Study the drawing (mm; zero at the part's minimum x, y, z) and answer. Round coordinates to 2 decimals unless told otherwise and drop trailing zeros. Order: outer loops, then holes, each group sorted by start corner. A loop starts at its lowest first (then second) coordinate and runs counter-clockwise, first axis right, second up. Notation, with made-up numbers: (-15.5, 6.5) - (14.5, 6.5) arc R23 cw to (14.5, 32.5) - close; hole circle Ø5 at (33.5, 1). An arc over 180 degrees is marked (long way). Put each result on its own line as item: value. Start each with the question number.
Q1. Find the intervals of material crossed by line 1 along X through (y, z) = (1.85, 88) (3 decimals); line 2 along Z through (x, y) = (12, 0.85) (3 decimals); line 3 along Z through (x, y) = (73.3, 2.05), in increasing order. Write a range as from..to.
Q2. This flat-tipped pin is pushed along its axis until it touches: pin 1 Ø2.5 at (x, z) = (73.3, 70) entering from +Y. Where does it stop, or does it pass through?
Q3. Section B-B on x = 73.3 is taken. Give the vertices of the cut face in (y, z), then the cut area to 3 significant figures.
Q4. Section A-A on z = 17.6 is taken. Give the vertices of the cut face in (x, y).
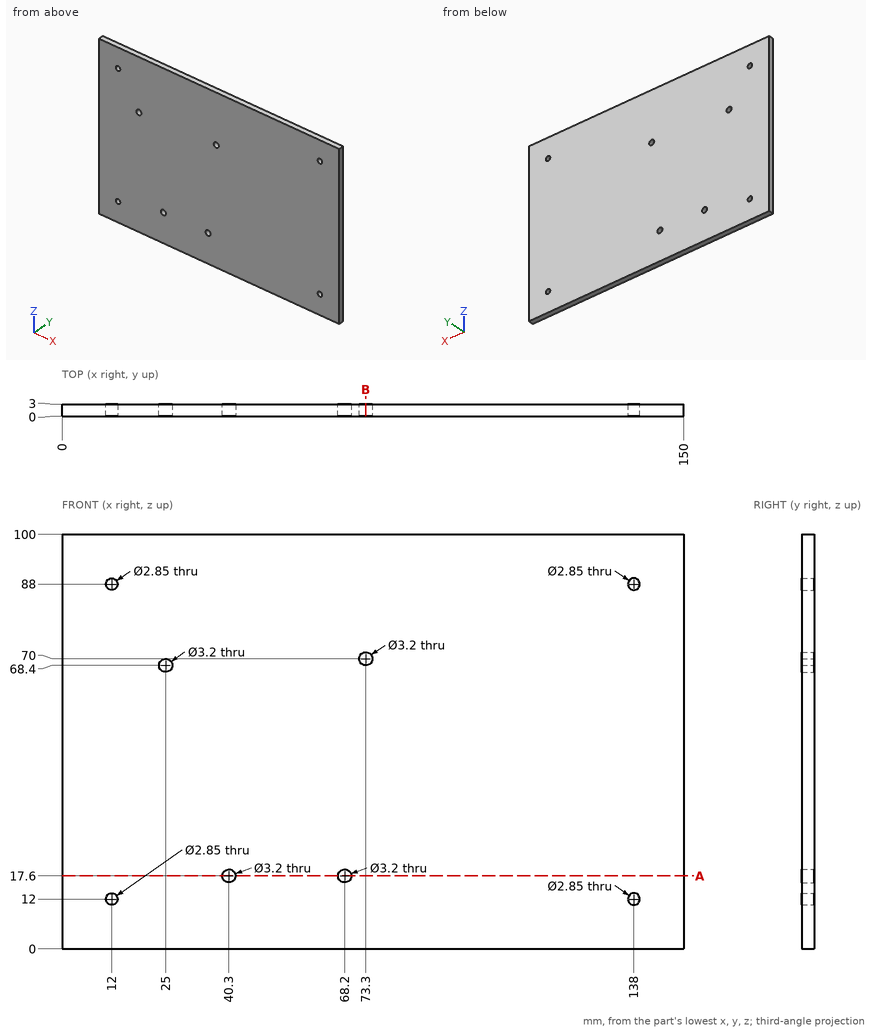
Findings:
1. line 1: 0..10.575, 13.425..136.575, 139.425..150
1. line 2: 0..10.575, 13.425..86.575, 89.425..100
1. line 3: 0..68.4, 71.6..100
2. pin 1: through
3. outline: (0, 0) - (3, 0) - (3, 68.4) - (0, 68.4) - close; (0, 71.6) - (3, 71.6) - (3, 100) - (0, 100) - close
3. area: 290 mm2
4. outline: (0, 0) - (38.7, 0) - (38.7, 3) - (0, 3) - close; (41.9, 0) - (66.6, 0) - (66.6, 3) - (41.9, 3) - close; (69.8, 0) - (150, 0) - (150, 3) - (69.8, 3) - close
